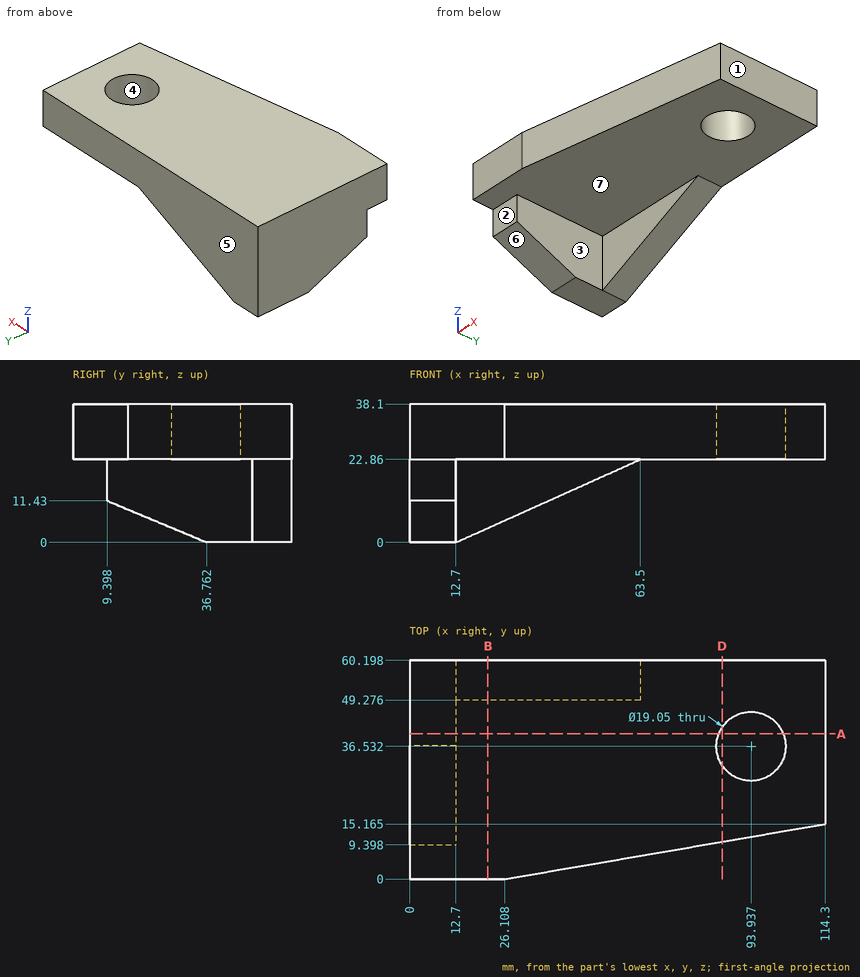
Answer from the drawing. Dimensions are ordinates in mm from the lowest x, y and z of the part. A direction names the side the tool comes from. Round coordinates to 2 decimals unless told otherwise and drop trailing zeros. Write each loop counter-clockwise with the first axis right and the second up, starting at its lowest first coordinate (ties: lowest second). Pieces come first, ordered by that corner, then holes.
1. Straight lines are drawn through the part: L1, parallel to X at y = 46.5, z = 6; L2, parallel to Z at x = 31.5, y = 45.5; L3, parallel to X at y = 31, z = 26.5 (1 decimal). For each, find the intervals that lie inside material, in ascending order.
2. Given pin 1 Ø1 at (x, y) = (67.5, 52.5) entering from -Z; pin 2 Ø10 at (x, z) = (69.5, 26.5) entering from -Y; pin 3 Ø18.5 at (x, z) = (49, 11.5) entering from -Y, each flat-ended and moving along its own axis, determine where each tip first touches the part or whether it passes through.
3. The part is cut by section D-D, the plane x = 86. Determine the outline of the cut face in (y, z).
4. The part is cut by section A-A, the plane y = 40. Determine the outline of the cut face in (x, z).
5. Which of the six approach directions +Z, -Z, +X, -X, +Y, -Y give full straight-line access (tool end or side, diameter ignored) to the marked faces 1, 2 and 3?
6. Determine the mould class of the marked faces 4, 5, 6 and 7 for opening direction Y: pulls with the +Y half, pulls with the -Y half, needs draft (parallel to the pull), parting line crosses it, or undercut.
7. The part is cut by section B-B, the plane x = 21.5. Determine the outline of the cut face in (y, z), then the cut area to 3 significant figures.
Values:
1. L1: x = 0 to 12.7
1. L2: z = 22.86 to 38.1
1. L3: x = 0 to 86.2, 101.7 to 114.3
2. pin 1: stops at z = 22.86
2. pin 2: stops at y = 6.6
2. pin 3: stops at y = 49.28
3. outline: (10.3, 22.86) - (31.27, 22.86) - (31.27, 38.1) - (10.3, 38.1) - close; (41.8, 22.86) - (60.2, 22.86) - (60.2, 38.1) - (41.8, 38.1) - close
4. outline: (0, 0) - (12.7, 0) - (12.7, 22.86) - (85.07, 22.86) - (85.07, 38.1) - (0, 38.1) - close; (102.81, 22.86) - (114.3, 22.86) - (114.3, 38.1) - (102.81, 38.1) - close
5. face 1: +Z, -Z, +X, +Y, -Y
5. face 2: -Z, +X, -X, -Y
5. face 3: -Z, +X, -Y
6. face 4: undercut
6. face 5: pulls with the +Y half
6. face 6: pulls with the -Y half
6. face 7: needs draft
7. outline: (0, 22.86) - (49.28, 22.86) - (49.28, 3.96) - (60.2, 3.96) - (60.2, 38.1) - (0, 38.1) - close
7. area: 1,120 mm2
